For this review, take the finished solid that the model builds, in its own axes (mm). Face numbers are marked on the shaded views. A direction names the side the tool comes from. Round coordinates to 2 decimals unless told otherwise and drop trailing zeros. Loops run counter-clockwise (first coordinate to the right, second up) from the corner with the lowest first, then second, coordinate; pieces in that order, holes last.
1. To check wall thickness, follow line 1 along Z through (x, y) = (20.5, -8.75); line 2 along Y through (x, z) = (29.5, 3.25); line 3 along X through (y, z) = (-16.25, 3.75). State the ranges of each line that lie inside material, in increasing order.
2. Consider section A-A on x = 18.5. State the section outline as (y, z) points.
3. Consider section C-C on z = -8.25. State the section outline as (x, y) points.
4. Draft analysis for pull direction X (two halves, no side actions). For the marked faces 5, 6 and 7, state which applies: released by +X, released by -X, zero draft, split by the parting line, or undercut.
5. Consider section B-B on y = -3. State the section outline as (x, z) points, then the cut area to 3 significant figures.
6. Consider section D-D on x = -13.5. State the section outline as (y, z) points, then the cut area to 3 significant figures.
7. Clearance check with flat-ended pins moving along their axes: pin 1 Ø3 at (y, z) = (-10, -4) entering from +X; pin 2 Ø12 at (x, z) = (31.5, -12.5) entering from -Y; pin 3 Ø10 at (x, y) = (-9.5, -19.5) entering from +Z. State where each tip first meets the part, or that it passes through.
8. Tool access review of the marked faces 1, 2, 3 and 4: name each direction out of +Z, -Z, +X, -X, +Y, -Y from which nothing blocks a thin tool from reaching the whole face with its end or side.
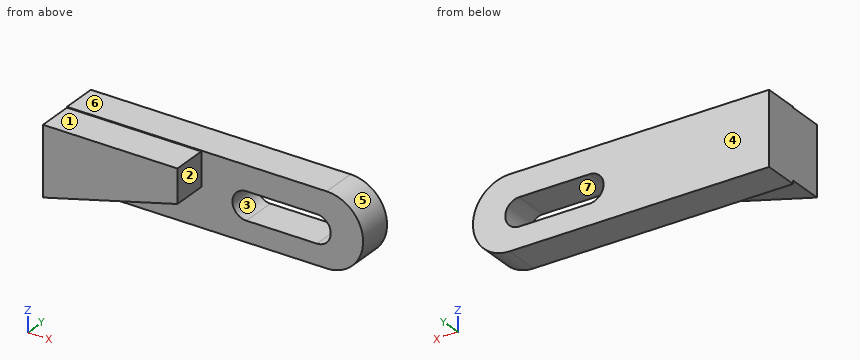
from build123d import *

# Parameters (mm, degrees)
F1_DEPTH = 25.4
F3_DEPTH = 12.7


with BuildPart() as f1:
    # F0 (on Front) → F1 (new body)
    with BuildSketch(Plane.XZ):
        Polygon((-9.248863, 8.514826), (-57.401668, 8.514826), (-57.401668, -16.148807), (-9.248863, -3.523376), align=None)
    extrude(amount=F1_DEPTH)

    # F2 (on Front) → F3 (join)
    with BuildSketch(Plane.XZ):
        with BuildLine():
            Line((35.674185, 8.808441), (-57.401668, 8.808441))
            Line((-57.401668, 8.808441), (-57.401668, -17.323267))
            Line((-57.401668, -17.323267), (35.674185, -17.323267))
            ThreePointArc((35.674185, -17.323267), (48.740038, -4.257413), (35.674185, 8.808441))
        make_face()
        with BuildLine():
            ThreePointArc((6.899945, -9.982899), (1.908496, -4.991449), (6.899945, 0))
            Line((6.899945, 0), (32.150805, 0))
            ThreePointArc((32.150805, 0), (37.142254, -4.991449), (32.150805, -9.982899))
            Line((32.150805, -9.982899), (6.899945, -9.982899))
        make_face(mode=Mode.SUBTRACT)
    extrude(amount=F3_DEPTH)


solid = f1.part
Resolved:
1. line 1: z = -17.32 to -9.98, 0 to 8.81
1. line 2: y = -12.7 to 0
1. line 3: x = -57.4 to -9.25
2. outline: (-12.7, -17.32) - (0, -17.32) - (0, -9.98) - (-12.7, -9.98) - close; (-12.7, 0) - (0, 0) - (0, 8.81) - (-12.7, 8.81) - close
3. outline: (-57.4, -25.4) - (-27.28, -25.4) - (-27.28, -12.7) - (3.12, -12.7) - (3.12, 0) - (-57.4, 0) - close; (35.93, -12.7) - (48.12, -12.7) - (48.12, 0) - (35.93, 0) - close
4. face 5: released by +X
4. face 6: zero draft
4. face 7: undercut
5. outline: (-57.4, -17.32) - (35.67, -17.32) arc R13.07 ccw to (35.67, 8.81) - (-57.4, 8.81) - close; hole (6.9, -9.98) - (32.15, -9.98) arc R4.99 ccw to (32.15, 0) - (6.9, 0) arc R4.99 ccw to start
5. area: 2,370 mm2
6. outline: (-25.4, -4.64) - (-12.7, -4.64) - (-12.7, -17.32) - (0, -17.32) - (0, 8.81) - (-12.7, 8.81) - (-12.7, 8.51) - (-25.4, 8.51) - close
6. area: 499 mm2
7. pin 1: stops at x = 48.74
7. pin 2: stops at y = -12.7
7. pin 3: stops at z = 8.51
8. face 1: +Z, +X, -X, -Y
8. face 2: +Z, -Z, +X, -Y
8. face 3: +Y, -Y
8. face 4: +Z, -Z, +X, -X, +Y
